from build123d import *

# Parameters (mm, degrees)
BOSS_EXTRUDE1_DEPTH                                 = 8
SKETCH2_R                                           = 17.5
SKETCH2_R_2                                         = 12.5
CUT_EXTRUDE1_DEPTH                                  = 9
SKETCH3_R                                           = 1.6
CUT_EXTRUDE2_DEPTH                                  = 9
SKETCH4_R                                           = 2.05
CUT_EXTRUDE3_DEPTH                                  = 9
CUT_EXTRUDE4_DEPTH                                  = 9
SKETCH6_R                                           = 1.6
SKETCH6_R_2                                         = 2.5
CUT_EXTRUDE5_DEPTH                                  = 9
SKETCH7_R                                           = 21
CUT_EXTRUDE6_DEPTH                                  = 7
CSK_FOR_M4_COUNTERSUNK_FLAT_HEAD_SCREW1_D           = 4.1
CSK_FOR_M4_COUNTERSUNK_FLAT_HEAD_SCREW1_CSINK_D     = 9.1
CSK_FOR_M4_COUNTERSUNK_FLAT_HEAD_SCREW1_CSINK_ANGLE = 90
CUT_EXTRUDE7_DEPTH                                  = 9


with BuildPart() as part:
    # Sketch1 → Boss-Extrude1 (new body)
    with BuildSketch(Plane(origin=(0, 0, 0), x_dir=(1, 0, 0), z_dir=(0, 1, 0))):
        with BuildLine():
            Line((-144, 39), (0, 39))
            ThreePointArc((0, 39), (39, 0), (0, -39))
            Line((0, -39), (-144, -39))
            ThreePointArc((-144, -39), (-183, 0), (-144, 39))
        make_face()
    extrude(amount=BOSS_EXTRUDE1_DEPTH)

    # Sketch2 → Cut-Extrude1 (cut, through all)
    with BuildSketch(Plane(origin=(0, 8, 0), x_dir=(1, 0, 0), z_dir=(0, 1, 0))):
        with Locations((-7.5, 0)):
            Circle(SKETCH2_R)
        with Locations((-150, 0)):
            Circle(SKETCH2_R_2)
    extrude(amount=-CUT_EXTRUDE1_DEPTH, mode=Mode.SUBTRACT)

    # Sketch3 → Cut-Extrude2 (cut, through all)
    with BuildSketch(Plane(origin=(0, 8, 0), x_dir=(1, 0, 0), z_dir=(0, 1, 0))):
        with Locations((-165.5, 15.5)):
            Circle(SKETCH3_R)
        with Locations((-134.5, 15.5)):
            Circle(SKETCH3_R)
        with Locations((-134.5, -15.5)):
            Circle(SKETCH3_R)
        with Locations((-165.5, -15.5)):
            Circle(SKETCH3_R)
    extrude(amount=-CUT_EXTRUDE2_DEPTH, mode=Mode.SUBTRACT)

    # Sketch4 → Cut-Extrude3 (cut, through all)
    with BuildSketch(Plane(origin=(0, 8, 0), x_dir=(1, 0, 0), z_dir=(0, 1, 0))):
        with Locations((-159.75, 27.279800219)):
            Circle(SKETCH4_R)
        with Locations((-175.5, 0)):
            Circle(SKETCH4_R)
        with Locations((-159.75, -27.279800219)):
            Circle(SKETCH4_R)
        with Locations((20.247809705, 24.130399958)):
            Circle(SKETCH4_R)
        with Locations((31.5, 0)):
            Circle(SKETCH4_R)
        with Locations((20.247809705, -24.130399958)):
            Circle(SKETCH4_R)
        with Locations((-99, 31.5)):
            Circle(SKETCH4_R)
        with Locations((-39, 31.5)):
            Circle(SKETCH4_R)
        with Locations((-39, -31.5)):
            Circle(SKETCH4_R)
        with Locations((-99, -31.5)):
            Circle(SKETCH4_R)
    extrude(amount=-CUT_EXTRUDE3_DEPTH, mode=Mode.SUBTRACT)

    # Sketch5 → Cut-Extrude4 (cut, through all)
    with BuildSketch(Plane(origin=(0, 8, 0), x_dir=(1, 0, 0), z_dir=(0, 1, 0))):
        with BuildLine():
            Line((-76.5, -25), (-76.5, -13))
            ThreePointArc((-76.5, -13), (-74, -10.5), (-71.5, -13))
            Line((-71.5, -13), (-71.5, -25))
            ThreePointArc((-71.5, -25), (-74, -27.5), (-76.5, -25))
        make_face()
        with BuildLine():
            Line((-71.5, 25), (-71.5, 13))
            ThreePointArc((-71.5, 13), (-74, 10.5), (-76.5, 13))
            Line((-76.5, 13), (-76.5, 25))
            ThreePointArc((-76.5, 25), (-74, 27.5), (-71.5, 25))
        make_face()
    extrude(amount=-CUT_EXTRUDE4_DEPTH, mode=Mode.SUBTRACT)

    # Sketch6 → Cut-Extrude5 (cut, through all)
    with BuildSketch(Plane(origin=(0, 8, 0), x_dir=(1, 0, 0), z_dir=(0, 1, 0))):
        with Locations((-48, -5)):
            Circle(SKETCH6_R)
        with Locations((-56.388002132, -9.459979846)):
            Circle(SKETCH6_R)
        with Locations((-59.5, 6)):
            Circle(SKETCH6_R_2)
    extrude(amount=-CUT_EXTRUDE5_DEPTH, mode=Mode.SUBTRACT)

    # Sketch7 → Cut-Extrude6 (cut)
    with BuildSketch(Plane(origin=(0, 8, 0), x_dir=(1, 0, 0), z_dir=(0, 1, 0))):
        with Locations((-7.5, 0)):
            Circle(SKETCH7_R)
    extrude(amount=-CUT_EXTRUDE6_DEPTH, mode=Mode.SUBTRACT)

    # CSK for M4 Countersunk Flat Head Screw1 (through all)
    with Locations(Plane(origin=(-159.75, 0, 27.279800219), x_dir=(0, 0, -1), z_dir=(0, -1, 0))):
        with Locations((0, 0), (27.279800219, -15.75), (54.559600438, 0), (-4.220199781, 60.75), (58.779800219, 60.75), (-4.220199781, 120.75), (58.779800219, 120.75), (3.149400261, 179.997809705), (27.279800219, 191.25), (51.410200177, 179.997809705)):
            CounterSinkHole(CSK_FOR_M4_COUNTERSUNK_FLAT_HEAD_SCREW1_D / 2, CSK_FOR_M4_COUNTERSUNK_FLAT_HEAD_SCREW1_CSINK_D / 2, counter_sink_angle=CSK_FOR_M4_COUNTERSUNK_FLAT_HEAD_SCREW1_CSINK_ANGLE)

    # Sketch9 → Cut-Extrude7 (cut, through all)
    with BuildSketch(Plane(origin=(0, 8, 0), x_dir=(1, 0, 0), z_dir=(0, 1, 0))):
        with BuildLine():
            Line((-122, -6), (-122, 6))
            ThreePointArc((-122, 6), (-119.2, 8.8), (-116.4, 6))
            Line((-116.4, 6), (-116.4, -6))
            ThreePointArc((-116.4, -6), (-119.2, -8.8), (-122, -6))
        make_face()
    extrude(amount=-CUT_EXTRUDE7_DEPTH, mode=Mode.SUBTRACT)


solid = part.part
The model under review builds one solid part; all positions refer to its coordinate system, in mm. A direction names the side the tool comes from. Give positions to 0.01 mm unless a question says otherwise; leave off trailing zeros. Order: outer loops, then holes, each group sorted by start corner. A loop starts at its lowest first (then second) coordinate and runs counter-clockwise, first axis right, second up. Notation, with made-up numbers: M 29.5,61.25 L 65.5,61.25 A19 cw 65.5,82.25 Z; hole C 38,56 d2. An arc over 180 degrees is marked long. Use one line per item in the form item = value. Start each with the question number.
Item 1: We need section B-B on x = -119.2. Give the boundary of the cut face in (y, z), plus the area to 3 significant figures.
Item 2: For faces 5 (the flat face through (-122, 4, 0)), 6 (the flat face through (-15, 1, -16)), 7 (the flat face through (-70, 0, -1)), list the 3-axis set-ups (+Z, -Z, +X, -X, +Y, -Y) from which the entire face can be reached by the end or side of a thin tool; tool diameter is ignored.
Item 3: We need section A-A on x = -39. Give the boundary of the cut face in (y, z), plus the area to 3 significant figures.
Item 4: The part is to be moulded in two halves that separate along Z. For faces 1 (the cylindrical face through (38.99, 3.94, -0.86)), 2 (the cylindrical face through (-37.9, 5.29, 29.77)), 3 (the flat face through (-71, 4, 39)), 4 (the cylindrical face through (0.575, 0.507, 15.526)), say which applies: pulls with the +Z half, pulls with the -Z half, needs draft (parallel to the pull), parting line crosses it, or undercut.
Item 5: To check wall thickness, follow line 1 along X through (y, z) = (0.5, 4.5); line 2 along Z through (x, y) = (-134.5, 2.75); line 3 along Z through (x, y) = (-48, 5.25). State the ranges of each line that lie inside material, in increasing order. Write a range as from..to.
Item 6: We need section C-C on x = -175.5. Give the boundary of the cut face in (y, z), plus the area to 3 significant figures.
Item 7: Insertion check: pin 1 Ø4 at (x, z) = (-56.39, 9.46) entering from -Y; pin 2 Ø5.5 at (x, z) = (-159.75, 27.28) entering from -Y; pin 3 Ø2.5 at (y, z) = (5.5, 1.5) entering from -X; pin 4 Ø4 at (y, z) = (2.5, -22) entering from +X. Each pin has a flat end and moves straight along its axis. Give the tip position at first contact, or say it passes through.
Item 8: We need section D-D on y = 3.75. Give the number of separate pieces and of enclosed holes in the cut face, plus the area to 3 significant figures.
Completed:
q1.outline = M 0,-39 L 8,-39 L 8,-8.8 L 0,-8.8 Z; M 0,8.8 L 8,8.8 L 8,39 L 0,39 Z
q1.area = 483 mm²
q2.face_5 = +Y, -Y
q2.face_6 = +Y
q2.face_7 = +Z, -Z, +X, -X, -Y
q3.outline = M 0,-39 L 8,-39 L 8,-33.55 L 2.5,-33.55 L 0,-36.05 Z; M 0,-26.95 L 2.5,-29.45 L 8,-29.45 L 8,29.45 L 2.5,29.45 L 0,26.95 Z; M 0,36.05 L 2.5,33.55 L 8,33.55 L 8,39 L 0,39 Z
q3.area = 546 mm²
q4.face_1 = parting line crosses it
q4.face_2 = undercut
q4.face_3 = pulls with the +Z half
q4.face_4 = undercut
q5.line_1 = -182.74..-161.66, -138.34..-122, -116.4..-49.52, -46.48..-24.41, 9.41..38.74
q5.line_2 = -39..-17.1, -13.9..13.9, 17.1..39
q5.line_3 = -39..3.4, 6.6..39
q6.outline = M 0,-22.99 L 8,-22.99 L 8,-2.05 L 2.5,-2.05 L 0,-4.55 Z; M 0,4.55 L 2.5,2.05 L 8,2.05 L 8,22.99 L 0,22.99 Z
q6.area = 329 mm²
q7.pin_1 = 0
q7.pin_2 = 1.8
q7.pin_3 = -183
q7.pin_4 = 33.48
q8.separate_pieces = 1
q8.enclosed_holes = 22
q8.area = 13,700 mm²
